Geometry: final body of the model. Coordinates: model frame, mm. A direction names the side the tool comes from. Give positions to 0.01 mm unless a question says otherwise; leave off trailing zeros. Write each loop counter-clockwise with the first axis right and the second up, starting at its lowest first coordinate (ties: lowest second). Pieces come first, ordered by that corner, then holes. Notation, with made-up numbers: M 18,16 L 51,16 A20 cw 51,31 Z; hole C 50,77 d10. An arc over 180 degrees is marked long. Answer as a JSON object with one key per item and string values.
from build123d import *

# Parameters (mm, degrees)
BOSS_EXTRU_1_DEPTH      = 240
ESQUISSE2_R             = 44.45
ENL_V_MAT_EXTRU_1_DEPTH = 78
ESQUISSE3_R             = 28.575
ENL_V_MAT_EXTRU_2_DEPTH = 205.284115878
BOSS_EXTRU_4_DEPTH      = 33
ESQUISSE8_W             = 33
ESQUISSE8_H             = 90
ENL_V_MAT_EXTRU_4_DEPTH = 19
ENL_V_MAT_EXTRU_4_DRAFT = -5
ENL_V_MAT_EXTRU_5_DEPTH = 13


with BuildPart() as part:
    # Esquisse1 → Boss.-Extru.1 (new body)
    with BuildSketch(Plane.XY):
        with BuildLine():
            Line((0, -86), (0, 88))
            ThreePointArc((0, 88), (-62.225396744, 62.225396744), (-88, 0))
            Line((-88, 0), (-88, -43.853430349))
            Line((-88, -43.853430349), (-13, -86))
            Line((-13, -86), (0, -86))
        make_face()
    extrude(amount=BOSS_EXTRU_1_DEPTH)

    # Esquisse2 → Enlèv. mat.-Extru.1 (cut)
    with BuildSketch(Plane.XY.offset(240)):
        Circle(ESQUISSE2_R)
    extrude(amount=-ENL_V_MAT_EXTRU_1_DEPTH, mode=Mode.SUBTRACT)

    # Esquisse3 → Enlèv. mat.-Extru.2 (cut, through all)
    with BuildSketch(Plane.XY.offset(162)):
        Circle(ESQUISSE3_R)
    extrude(amount=-ENL_V_MAT_EXTRU_2_DEPTH, mode=Mode.SUBTRACT)

    # Esquisse7 → Boss.-Extru.4 (add)
    with BuildSketch(Plane.XY.offset(240)):
        with BuildLine():
            Line((-64.719928969, 0), (-40.188548434, 31.398735242))
            Line((-40.188548434, 31.398735242), (-14.235687992, 64.616881796))
            Line((-14.235687992, 64.616881796), (-34.918120487, 80.775769025))
            ThreePointArc((-34.918120487, 80.775769025), (-68.534051615, 55.20039646), (-86.360508015, 16.907473358))
            Line((-86.360508015, 16.907473358), (-64.719928969, 0))
        make_face()
    extrude(amount=BOSS_EXTRU_4_DEPTH)


with BuildPart() as enl_v_mat_extru_4_tool:
    # Esquisse8 → Enlèv. mat.-Extru.4 (with draft: the straight prism first)
    with BuildSketch(Plane(origin=(0, 0, 0), x_dir=(0, 0, -1), z_dir=(1, 0, 0))):
        with Locations((-54.5, 49.335999727)):
            Rectangle(ESQUISSE8_W, ESQUISSE8_H)
    extrude(amount=-ENL_V_MAT_EXTRU_4_DEPTH)
    # Enlèv. mat.-Extru.4: the draft: its side faces are tilted about the plane it starts from
    enl_v_mat_extru_4_sides = [enl_v_mat_extru_4_tool.faces().sort_by_distance(p)[0] for p in [
        (-9.5, 49.335999727, 71),
        (-9.5, 4.335999727, 54.5),
        (-9.5, 49.335999727, 38),
        (-9.5, 94.335999727, 54.5),
    ]]
    draft(enl_v_mat_extru_4_sides, Plane(origin=(0, 0, 0), x_dir=(0, 0, -1), z_dir=(1, 0, 0)), ENL_V_MAT_EXTRU_4_DRAFT)


with BuildPart() as part_1:
    add(part.part)

    # Enlèv. mat.-Extru.4: cut by enl_v_mat_extru_4_tool
    add(enl_v_mat_extru_4_tool.part, mode=Mode.SUBTRACT)

    # Esquisse9 → Enlèv. mat.-Extru.5 (cut)
    with BuildSketch(Plane(origin=(0, 0, 0), x_dir=(0, 0, -1), z_dir=(1, 0, 0))):
        with BuildLine():
            Line((-113, -49), (0, -49))
            Line((0, -49), (0, -71))
            Line((0, -71), (-113, -71))
            ThreePointArc((-113, -71), (-124, -60), (-113, -49))
        make_face()
    extrude(amount=-ENL_V_MAT_EXTRU_5_DEPTH, mode=Mode.SUBTRACT)


solid = part_1.part
1) Contact query for flat-ended pins moving along their axis: P1, Ø12, axis at x = -27, z = 39.5, coming from the -Y side; P2, Ø6, axis at x = -38, z = 73, coming from the -Y side; P3, Ø22, axis at x = -21.5, y = -12.5, coming from the +Z side. Output: stop coordinate, or through.
Geometry check:
{"P1": "stops at y = -81.5", "P2": "stops at y = -73.64", "P3": "stops at z = 162"}
2) Cut plane D-D on z = 50. Return loops of the section in (x, y) (3 decimals).
Geometry check:
{"outline": "M -88,-43.853 L -13,-86 L 0,-86 L 0,-71 L -13,-71 L -13,-49 L 0,-49 L 0,-28.575 A28.575 cw -19,21.343 L -19,85.924 A88 ccw -88,0 Z"}
3) Cut plane A-A on z = 235. Return loops of the section in (x, y), and give its area (3 significant figures).
Geometry check:
{"outline": "M -88,-43.85 L -13,-86 L 0,-86 L 0,-44.45 A44.45 cw 0,44.45 L 0,88 A88 ccw -88,0 Z", "area": "8,970 mm2"}
4) Line query: line 1 (Z direction, x = -65, y = -0.5); line 2 (Y direction, x = -39, z = 218); line 3 (Y direction, x = -23.5, z = 86.5). Output: solid intervals per line, ascending. Write a range as from..to.
Geometry check:
{"line 1": "z = 0..240", "line 2": "y = -71.39..-21.33, 21.33..78.89", "line 3": "y = -80.1..-16.26, 16.26..84.8"}
5) Set-up query: faces 1 (the flat face through (-75.69, 8.57, 256.27)), 2 (the flat face through (-9.37, 54.2, 38.82)), 3 (the flat face through (-6, -71, 56)), 4 (the flat face through (-32, 1, 162)). Return all of +Z, -Z, +X, -X, +Y, -Y with unobstructed straight access to the full face (end or side cutting, diameter ignored); none if empty.
Geometry check:
{"face 1": "+Z, -X, -Y", "face 2": "+X, +Y", "face 3": "-Z, +X", "face 4": "+Z, +X"}
6) Cut plane C-C on y = 37.5. Return loops of the section in (x, z), and give its area (3 significant figures).
Geometry check:
{"outline": "M -79.61,0 L 0,0 L 0,38 L -19,39.66 L -19,69.34 L 0,71 L 0,162 L -23.87,162 L -23.87,240 L -35.42,240 L -35.42,273 L -79.61,273 Z", "area": "18,100 mm2"}
7) Cut plane B-B on x = -32. Return loops of the section in (y, z).
Geometry check:
{"outline": "M -75.32,0 L 81.98,0 L 81.98,240 L 78.5,240 L 78.5,273 L 41.88,273 L 41.88,240 L 30.85,240 L 30.85,162 L -30.85,162 L -30.85,240 L -75.32,240 Z"}
8) Pull-direction query (Y, two-part tool) for faces 5 (the flat face through (-51.025, -64.632, 118.32)), 6 (the flat face through (-6, -49, 57)), 7 (the flat face through (-88, -22, 118)); classes: pulls with the +Y half, pulls with the -Y half, needs draft (parallel to the pull), parting line crosses it, or undercut.
Geometry check:
{"face 5": "pulls with the -Y half", "face 6": "undercut", "face 7": "needs draft"}
